Source: CAD feature listing. Evaluate the final solid. Frame: model axes, mm. A direction names the side the tool comes from. Coordinates: 2 decimals unless noted, no trailing zeros. Loops run counter-clockwise (first coordinate to the right, second up) from the corner with the lowest first, then second, coordinate; pieces in that order, holes last. Notation, with made-up numbers: (-36.75, 25) -> (5.25, 25) arc R35 ccw to (5.25, 58) -> close; hole circle Ø11 at (-38, -8). An arc over 180 degrees is marked (long way). Answer as a JSON object with one key per item and string values. Group by question number.
from build123d import *

# Parameters (mm, degrees)
SKETCH_2_R          = 10
CUT_EXTRUDE_1_DEPTH = 10


with BuildPart() as part:
    # 草图1 → 旋转1 (revolve)
    with BuildSketch(Plane.XY, mode=Mode.PRIVATE) as revolve_1_sk:
        Polygon((-3, 33.921052632), (-9, 33.921052632), (-9, 29.921052632), (-40, 29.921052632), (-40, 33.921052632), (-45, 33.921052632), (-45, 32.921052632), (-47.75, 32.921052632), (-47.75, 20.921052632), (-45, 20.921052632), (-45, 19.921052632), (-40, 19.921052632), (-40, 23.921052632), (-9, 23.921052632), (-9, 19.921052632), (-9, 14.721052632), (-3, 14.721052632), align=None)
    revolve(revolve_1_sk.sketch.rotate(Axis((0, 0, 0), (0, 1, 0)), 270), axis=Axis((0, 0, 0), (0, 1, 0)))

    # 草图2 → 切除-拉伸1 (cut)
    with BuildSketch(Plane.XZ.offset(-23.921052632)):
        with Locations(Location((0, 24, 0), (0, 0, 270))):
            Circle(SKETCH_2_R)
        with Locations(Location((22.825356391, 7.416407865, 0), (0, 0, 270))):
            Circle(SKETCH_2_R)
        with Locations(Location((14.106846055, -19.416407865, 0), (0, 0, 270))):
            Circle(SKETCH_2_R)
        with Locations(Location((-14.106846055, -19.416407865, 0), (0, 0, 270))):
            Circle(SKETCH_2_R)
        with Locations(Location((-22.825356391, 7.416407865, 0), (0, 0, 270))):
            Circle(SKETCH_2_R)
    extrude(amount=-CUT_EXTRUDE_1_DEPTH, mode=Mode.SUBTRACT)


solid = part.part
1. Section query A-A on z = 24. Return loops of the section in (x, y), then the cut area to 3 significant figures.
2. Mould query, pull axis Z, two halves, no side actions, for faces 4 (the face through (39.05, 21.95, 8.67)), 5 (the face through (4, 14.721, 0)), 6 (the face through (-0.6, 23.921, 9.4)), 7 (the face through (17.235, 33.414, -41.569)). Classes: pulls with the +Z half, pulls with the -Z half, needs draft (parallel to the pull), parting line crosses it, or undercut.
3. Ray query, L1, parallel to X at y = 32.5, z = 0; L2, parallel to Z at x = -23, y = 26.5; L3, parallel to Z at x = -17.5, y = 26. Return the intervals inside material, ascending.
4. Section query D-D on x = 37. Return loops of the section in (y, z).
5. Pin query (flat end, axial travel): pin 1 Ø1.5 at (y, z) = (20, -22) entering from -X; pin 2 Ø4 at (x, z) = (-18, 31.5) entering from -Y; pin 3 Ø10 at (x, y) = (31.5, 17.5) entering from +Z; pin 4 Ø6 at (x, z) = (33, 31.5) entering from +Y. Return the tip coordinate at first contact, or that it passes through.
6. Section query C-C on z = -27. Return loops of the section in (x, y), then the cut area to 3 significant figures.
7. Section query B-B on y = 26.5. Return loops of the section in (x, z).
8. Reachability of faces 1 (the face through (17.235, 20.414, -41.569)), 2 (the face through (-0.9, 24.46, -2.86)), 3 (the face through (8, 29.921, 8)) from +Z, -Z, +X, -X, +Y, -Y: full face, straight path, thin tool, end or side. Return the list, or none.
Solved:
{
 "1": {"outline": "(-41.28, 20.92) -> (-38.07, 20.92) -> (-38.07, 19.92) -> (-32, 19.92) -> (-32, 23.92) -> (-10, 23.92) -> (-10, 29.92) -> (-32, 29.92) -> (-32, 33.92) -> (-38.07, 33.92) -> (-38.07, 32.92) -> (-41.28, 32.92) -> close; (10, 23.92) -> (32, 23.92) -> (32, 19.92) -> (38.07, 19.92) -> (38.07, 20.92) -> (41.28, 20.92) -> (41.28, 32.92) -> (38.07, 32.92) -> (38.07, 33.92) -> (32, 33.92) -> (32, 29.92) -> (10, 29.92) -> close", "area": "511 mm^2"},
 "2": {"face 4": "undercut", "face 5": "needs draft", "face 6": "undercut", "face 7": "parting line crosses it"},
 "3": {"L1": "-47.75 to -40, -9 to -3, 3 to 9, 40 to 47.75", "L2": "-41.85 to -23.99, -14.84 to -2.58, 17.41 to 41.85", "L3": "-44.43 to -28.82, -10.01 to -1.05, 15.88 to 44.43"},
 "4": {"outline": "(19.92, -25.61) -> (20.92, -25.61) -> (20.92, -30.18) -> (32.92, -30.18) -> (32.92, -25.61) -> (33.92, -25.61) -> (33.92, -15.2) -> (29.92, -15.2) -> (29.92, 15.2) -> (33.92, 15.2) -> (33.92, 25.61) -> (32.92, 25.61) -> (32.92, 30.18) -> (20.92, 30.18) -> (20.92, 25.61) -> (19.92, 25.61) -> (19.92, 15.2) -> (23.92, 15.2) -> (23.92, -15.2) -> (19.92, -15.2) -> close"},
 "5": {"pin 1": "x = -39.67", "pin 2": "y = 23.92", "pin 3": "z = 38.78", "pin 4": "y = 33.92"},
 "6": {"outline": "(-39.38, 20.92) -> (-36, 20.92) -> (-36, 19.92) -> (-29.51, 19.92) -> (-29.51, 23.92) -> (-20.63, 23.92) -> (-20.63, 29.92) -> (-29.51, 29.92) -> (-29.51, 33.92) -> (-36, 33.92) -> (-36, 32.92) -> (-39.38, 32.92) -> close; (-7.59, 23.92) -> (7.59, 23.92) -> (7.59, 29.92) -> (-7.59, 29.92) -> close; (20.63, 23.92) -> (29.51, 23.92) -> (29.51, 19.92) -> (36, 19.92) -> (36, 20.92) -> (39.38, 20.92) -> (39.38, 32.92) -> (36, 32.92) -> (36, 33.92) -> (29.51, 33.92) -> (29.51, 29.92) -> (20.63, 29.92) -> close", "area": "461 mm^2"},
 "7": {"outline": "circle Ø95.5 at (0, 0); hole circle Ø20 at (-22.83, 7.42); hole circle Ø20 at (-14.11, -19.42); hole circle Ø20 at (0, 24); hole circle Ø6 at (0, 0); hole circle Ø20 at (14.11, -19.42); hole circle Ø20 at (22.83, 7.42)"},
 "8": {"face 1": "-Y", "face 2": "+Y, -Y", "face 3": "+Y"}
}
